Check sheet for the modelled part. Datum: model origin and axes. Units: mm. Face numbers are marked on the shaded views. A direction names the side the tool comes from. Round coordinates to 2 decimals unless told otherwise and drop trailing zeros. Write each loop counter-clockwise with the first axis right and the second up, starting at its lowest first coordinate (ties: lowest second). Pieces come first, ordered by that corner, then holes. Notation, with made-up numbers: (88.5, 56.25) - (139.5, 56.25) arc R25 cw to (139.5, 80.25) - close; hole circle Ø10 at (-23.5, 6.25). An arc over 180 degrees is marked (long way). Answer as a JSON object with one key per item and string values. Group by question number.
Item 1: Gauge pin test, flat ends, axial feed: P1, Ø4, axis at y = 9, z = 2.5, coming from the -X side; P2, Ø5, axis at x = -5, y = 6, coming from the -Z side; P3, Ø4, axis at y = 7.5, z = -7, coming from the +X side. Record the tip position at first contact, or that the pin passes through.
Item 2: Thickness scan on line 1 (X direction, y = 9.5, z = 0); line 2 (Y direction, x = -0.75, z = -5.5); line 3 (X direction, y = 3.75, z = 5.25). Record the ranges inside material, lowest first.
Item 3: Set-up check for the marked faces 4 and 5: record each of +Z, -Z, +X, -X, +Y, -Y from which the full face is reachable in a straight line by a thin tool's end or side.
Item 4: Sectioned sample at A-A on z = 0. Record the boundary of the cut face in (x, y), plus the area to 3 significant figures.
Item 5: Release check for a two-part mould opening along X. For the marked faces 1, 2 and 3 record: pulls with the +X half, pulls with the -X half, needs draft (parallel to the pull), parting line crosses it, or undercut.
Item 6: Sectioned sample at B-B on y = 7.5. Record the boundary of the cut face in (x, z).
Item 7: Sectioned sample at C-C on y = 12.5. Record the boundary of the cut face in (x, z).
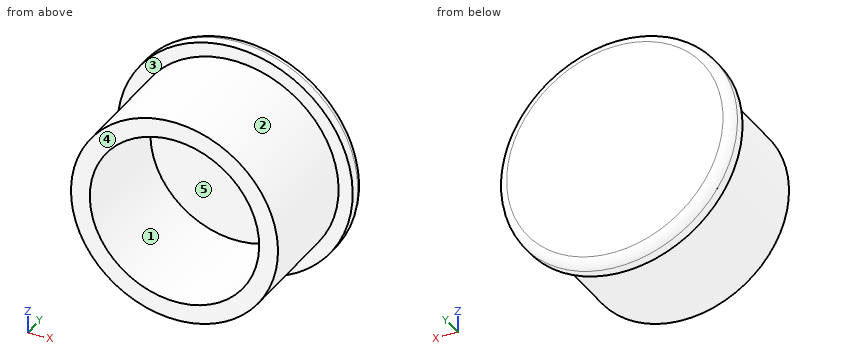
```python
from build123d import *

# Parameters (mm, degrees)
SKETCH2_R           = 11
SKETCH2_R_2         = 9
BOSS_EXTRUDE1_DEPTH = 12
SKETCH3_R           = 12.5
BOSS_EXTRUDE2_DEPTH = 2
FILLET1_R           = 1


with BuildPart() as part:
    # Sketch2 → Boss-Extrude1 (new body)
    with BuildSketch(Plane(origin=(0, 0, 0), x_dir=(1, 0, 0), z_dir=(0, 1, 0))):
        with Locations(Location((0, 0, 0), (0, 0, 270))):
            Circle(SKETCH2_R)
        with Locations(Location((0, 0, 0), (0, 0, 270))):
            Circle(SKETCH2_R_2, mode=Mode.SUBTRACT)
    extrude(amount=BOSS_EXTRUDE1_DEPTH)

    # Sketch3 → Boss-Extrude2 (add)
    with BuildSketch(Plane(origin=(0, 12, 0), x_dir=(1, 0, 0), z_dir=(0, 1, 0))):
        with Locations(Location((0, 0, 0), (0, 0, 270))):
            Circle(SKETCH3_R)
    extrude(amount=BOSS_EXTRUDE2_DEPTH)

    # Fillet1
    fillet1_edges = [part.edges().sort_by_distance(p)[0] for p in [
        (0, 14, -12.5),
    ]]
    fillet(fillet1_edges, radius=FILLET1_R)


solid = part.part
```
Completed:
{
 "1": {"P1": "x = -10.99", "P2": "z = -10.71", "P3": "x = 9.8"},
 "2": {"line 1": "-11 to -9, 9 to 11", "line 2": "12 to 14", "line 3": "-9.67 to -7.31, 7.31 to 9.67"},
 "3": {"face 4": "+Z, -Z, +X, -X, -Y", "face 5": "-Y"},
 "4": {"outline": "(-12.5, 12) - (-11, 12) - (-11, 0) - (-9, 0) - (-9, 12) - (9, 12) - (9, 0) - (11, 0) - (11, 12) - (12.5, 12) - (12.5, 13) arc R1 ccw to (11.5, 14) - (-11.5, 14) arc R1 ccw to (-12.5, 13) - close", "area": "97.6 mm²"},
 "5": {"face 1": "undercut", "face 2": "parting line crosses it", "face 3": "needs draft"},
 "6": {"outline": "circle Ø22 at (0, 0); hole circle Ø18 at (0, 0)"},
 "7": {"outline": "circle Ø25 at (0, 0)"}
}
